```python
from build123d import *

# Parameters (mm, degrees)
EXTRUDE_1_DEPTH     = 3
CUT_EXTRUDE_1_DEPTH = 3


with BuildPart() as part:
    # 스케치1 → 보스-돌출1 (new body)
    with BuildSketch(Plane(origin=(0, 0, 0), x_dir=(0, 0, -1), z_dir=(1, 0, 0))):
        Polygon((0, 0), (20, 0), (20, 290), (-20, 290), (-20, 248), (0, 248), align=None)
    extrude(amount=EXTRUDE_1_DEPTH)

    # 스케치2 → 컷-돌출1 (cut)
    with BuildSketch(Plane(origin=(3, 0, 0), x_dir=(0, 0, -1), z_dir=(1, 0, 0))):
        Polygon((10, 290), (20, 248), (20, 290), align=None)
    extrude(amount=-CUT_EXTRUDE_1_DEPTH, mode=Mode.SUBTRACT)


solid = part.part
```
The model under review builds one solid part; all positions refer to its coordinate system, in mm. Give positions to 0.01 mm unless a question says otherwise; leave off trailing zeros. Write each loop counter-clockwise with the first axis right and the second up, starting at its lowest first coordinate (ties: lowest second). Pieces come first, ordered by that corner, then holes. Notation, with made-up numbers: M 59.25,59 L 71.25,59 A20 ccw 71.25,97 Z; hole C -35.5,52 d8. An arc over 180 degrees is marked long. Answer in a Markdown table with one row per item.
Item 1: Add section A-A on x = 2.55. Give the boundary of the cut face in (y, z).
Check sheet entries:
| item | result |
|---|---|
| outline | M 0,-20 L 248,-20 L 290,-10 L 290,20 L 248,20 L 248,0 L 0,0 Z |
Item 2: Add section B-B on z = 16.5. Give the boundary of the cut face in (x, y), plus the area to 3 significant figures.
Check sheet entries:
| item | result |
|---|---|
| outline | M 0,248 L 3,248 L 3,290 L 0,290 Z |
| area | 126 mm2 |
Item 3: For P1, Ø0.9, axis at x = 2, y = 171.5, coming from the +Z side; P2, Ø1.5, axis at x = 2.5, z = 0.5, coming from the -Y side, all flat-tipped, find the tip position at first contact; note any pin that passes through.
Check sheet entries:
| item | result |
|---|---|
| P1 | z = 0 |
| P2 | y = 0 |
Item 4: For line 1 along Y through (x, z) = (2.5, 3.5); line 2 along Z through (x, y) = (1.65, 193.5); line 3 along Z through (x, y) = (1.8, 260), list the stretches that pass through material, from the lowest coordinate up.
Check sheet entries:
| item | result |
|---|---|
| line 1 | 248 to 290 |
| line 2 | -20 to 0 |
| line 3 | -17.14 to 20 |
Item 5: Add section C-C on y = 51. Give the boundary of the cut face in (x, z), plus the area to 3 significant figures.
Check sheet entries:
| item | result |
|---|---|
| outline | M 0,-20 L 3,-20 L 3,0 L 0,0 Z |
| area | 60.0 mm2 |
